from build123d import *

# Parameters (mm, degrees)
PAD005_DEPTH    = 7
SKETCH018_W     = 0.5
SKETCH018_H     = 0.5
PAD006_DEPTH    = 10
SKETCH019_W     = 3
SKETCH019_H     = 3
POCKET003_DEPTH = 0.1


with BuildPart() as part:
    # Sketch017 → Pad005 (new body)
    with BuildSketch(Plane.XY):
        with BuildLine():
            ThreePointArc((2.193171, -1.2), (0, 2.5), (-2.193171, -1.2))
            Line((-2.193171, -1.2), (2.193171, -1.2))
        make_face()
    extrude(amount=PAD005_DEPTH)

    # Sketch018 (on Face3 of Pad005) → Pad006 (join)
    with BuildSketch(Plane(origin=(0, 0, 0), x_dir=(1, 0, 0), z_dir=(0, 0, -1))):
        with Locations((-1.25, 0)):
            Rectangle(SKETCH018_W, SKETCH018_H)
        with Locations((1.25, 0)):
            Rectangle(SKETCH018_W, SKETCH018_H)
    extrude(amount=PAD006_DEPTH)

    # Sketch019 (on Face2 of Pad006) → Pocket003 (cut)
    with BuildSketch(Plane.XZ.offset(1.2)):
        with Locations((0, 4.5)):
            Rectangle(SKETCH019_W, SKETCH019_H)
    extrude(amount=-POCKET003_DEPTH, mode=Mode.SUBTRACT)


solid = part.part
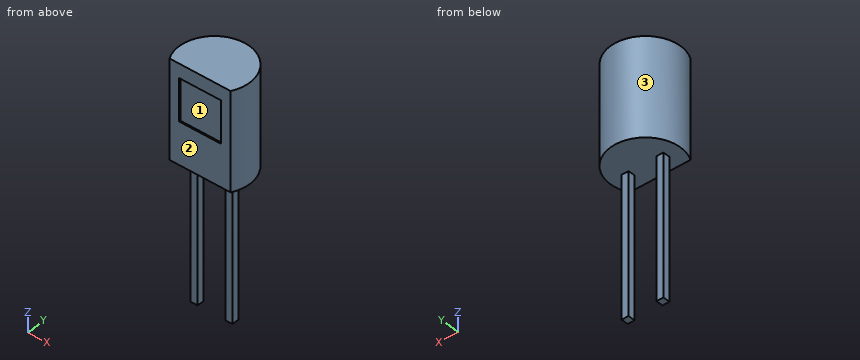
Model file for the job. Use its own axes, mm. Face numbers are marked on the shaded views. Give positions to 0.01 mm unless a question says otherwise; leave off trailing zeros. Order: outer loops, then holes, each group sorted by start corner. A loop starts at its lowest first (then second) coordinate and runs counter-clockwise, first axis right, second up. Notation, with made-up numbers: M 28,-37.75 L 63,-37.75 A22 cw 63,-28.75 Z; hole C 31.25,68 d8. An arc over 180 degrees is marked long. Put each result on its own line as item: value. Start each with the question number.
(1) Band-saw the part on A-A on z = -2. Give the cut face in (x, y), then the cut area to 3 significant figures.
(2) Pin check, flat tips, straight feed: pin 1 Ø0.6 at (y, z) = (0, -7) entering from +X; pin 2 Ø0.6 at (x, z) = (-1, -3) entering from +Y. Stop position of each tip, or through.
(3) Band-saw the part on D-D on z = 2.5. Give the cut face in (x, y), then the cut area to 3 significant figures.
(4) Band-saw the part on C-C on x = 0. Give the cut face in (y, z), then the cut area to 3 significant figures.
(5) Band-saw the part on B-B on y = 0. Give the cut face in (x, z).
(6) Drill centre lines: L1, parallel to Z at x = -0.05, y = -0.5; L2, parallel to Y at x = 1.1, z = -3.5; L3, parallel to Y at x = 0.7, z = 2.75. Where is each one in solid material? Low to high. Write a range as [from, to].
(7) Pull direction X, two halves, no side cores. Call the marked faces 1, 2 and 3: released by +X, released by -X, zero draft, split by the parting line, or undercut.
Results below:
1. outline: M -1.5,-0.25 L -1,-0.25 L -1,0.25 L -1.5,0.25 Z; M 1,-0.25 L 1.5,-0.25 L 1.5,0.25 L 1,0.25 Z
1. area: 0.500 mm2
2. pin 1: stops at x = 1.5
2. pin 2: stops at y = 0.25
3. outline: M -2.19,-1.2 L 2.19,-1.2 A2.5 ccw long Z
3. area: 15.6 mm2
4. outline: M -1.2,0 L 2.5,0 L 2.5,7 L -1.2,7 L -1.2,6 L -1.1,6 L -1.1,3 L -1.2,3 Z
4. area: 25.6 mm2
5. outline: M -2.5,0 L -1.5,0 L -1.5,-10 L -1,-10 L -1,0 L 1,0 L 1,-10 L 1.5,-10 L 1.5,0 L 2.5,0 L 2.5,7 L -2.5,7 Z
6. L1: z = [0, 7]
6. L2: y = [-0.25, 0.25]
6. L3: y = [-1.2, 2.4]
7. face 1: undercut
7. face 2: zero draft
7. face 3: split by the parting line
